Input: part model. Units: mm. Frame: model coordinates. Face numbers are marked on the shaded views. A direction names the side the tool comes from. Round coordinates to 2 decimals unless told otherwise and drop trailing zeros. Order: outer loops, then holes, each group sorted by start corner. A loop starts at its lowest first (then second) coordinate and runs counter-clockwise, first axis right, second up. Notation, with made-up numbers: (34, 55.5) -> (87, 55.5) arc R18 ccw to (87, 79.5) -> close; hole circle Ø5 at (-15, 30). An arc over 180 degrees is marked (long way). Answer as CSV lines item,"result". Start each with the question number.
1) First-contact query: P1, Ø1.2, axis at x = -6, z = -10.5, coming from the -Y side; P2, Ø2.5, axis at y = 9.5, z = -6, coming from the +X side; P3, Ø1, axis at x = -3.5, y = -1, coming from the -Z side. Flat tips, straight axial feed; report the tip coordinate or a pass-through.
2) Section query D-D, the plane z = 0.5. Output: boundary loops of the cut face in (x, y).
3) Access query for the marked faces 5 and 6. Directions: +Z, -Z, +X, -X, +Y, -Y. A direction counts if a zero-diameter tool reaches every point of the face in a straight line with its end or side. Return the directions, or none.
4) Section query B-B, the plane z = 6.5. Output: boundary loops of the cut face in (x, y), and give its area (3 significant figures).
5) Section query A-A, the plane z = 9. Output: boundary loops of the cut face in (x, y), and give its area (3 significant figures).
6) Section query C-C, the plane x = 7. Output: boundary loops of the cut face in (y, z), and give its area (3 significant figures).
7) Mould query, pull axis Z, two halves, no side actions, for the marked faces 1, 2, 3 and 4. Classes: +Z half, -Z half, draft (parallel to the pull), parting line (faces both ways), or undercut.
8) Line query: L1, parallel to Z at x = -13.9, y = 10; L2, parallel to X at y = 6.25, z = 3.75; L3, parallel to Z at x = -10.5, y = -0.75. Output: solid intervals per line, ascending.
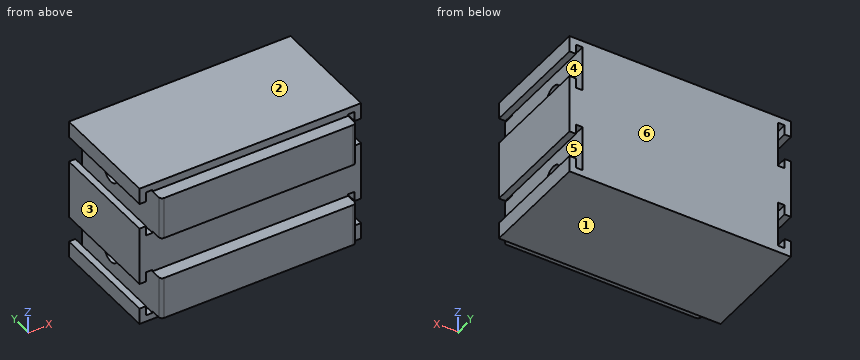
```python
from build123d import *

# Parameters (mm, degrees)
F0_W      = 34
F0_H      = 22
F1_DEPTH  = 17
F3_DEPTH  = 17.001
F4_W      = 30
F4_H      = 6.5
F5_DEPTH  = 2
F7_R      = 1.6
F8_DEPTH  = 5
F10_R     = 1.6
F11_DEPTH = 5
F12_R     = 0.5


with BuildPart() as f1:
    # F0 (on Front) → F1 (new body)
    with BuildSketch(Plane.XZ):
        Rectangle(F0_W, F0_H)
    extrude(amount=-F1_DEPTH)

    # F2 (on face) → F3 (cut, through all)
    with BuildSketch(Plane.XZ):
        Polygon((-16, 8.5), (-17, 8.5), (-17, 4.5), (-16, 4.5), (-16, 3), (-15, 3), (-15, 10), (-16, 10), align=None)
        Polygon((15, 10), (15, 3), (16, 3), (16, 4.5), (17, 4.5), (17, 8.5), (16, 8.5), (16, 10), align=None)
        Polygon((17, -4.5), (16, -4.5), (16, -3), (15, -3), (15, -10), (16, -10), (16, -8.5), (17, -8.5), align=None)
        Polygon((-17, -4.5), (-17, -8.5), (-16, -8.5), (-16, -10), (-15, -10), (-15, -3), (-16, -3), (-16, -4.5), align=None)
    extrude(amount=-F3_DEPTH, mode=Mode.SUBTRACT)

    # F4 (on face) → F5 (join)
    with BuildSketch(Plane.XZ):
        with Locations((0, 6.5)):
            Rectangle(F4_W, F4_H)
        with Locations((0, -6.5)):
            Rectangle(F4_W, F4_H)
    extrude(amount=F5_DEPTH)

    # F7 (on offset) → F8 (cut)
    with BuildSketch(Plane(origin=(-15, 0, 0), x_dir=(0, -1, 0), z_dir=(-1, 0, 0))):
        with Locations((-10, 6.5)):
            Circle(F7_R)
        with Locations((-10, -6.5)):
            Circle(F7_R)
    extrude(amount=-F8_DEPTH, mode=Mode.SUBTRACT)

    # F10 (on offset) → F11 (cut)
    with BuildSketch(Plane.YZ.offset(15)):
        with Locations((10, 6.5)):
            Circle(F10_R)
        with Locations((10, -6.5)):
            Circle(F10_R)
    extrude(amount=-F11_DEPTH, mode=Mode.SUBTRACT)

    # F12
    f12_edges = [f1.edges().sort_by_distance(p)[0] for p in [
        (15, -2, 6.5),
        (-15, -2, 6.5),
        (15, -2, -6.5),
        (-15, -2, -6.5),
    ]]
    fillet(f12_edges, radius=F12_R)


solid = f1.part
```
Findings:
1,P1,"stops at y = 0"
1,P2,"stops at x = 15"
1,P3,"stops at z = -9.75"
2,outline,"(-17, 0) -> (17, 0) -> (17, 17) -> (-17, 17) -> close"
3,face 5,"+Y, -Y"
3,face 6,"+Z, -Z, +X, -X, +Y"
4,outline,"(-15, -1.5) arc R0.5 ccw to (-14.5, -2) -> (14.5, -2) arc R0.5 ccw to (15, -1.5) -> (15, 8.4) -> (10, 8.4) -> (10, 11.6) -> (15, 11.6) -> (15, 17) -> (-15, 17) -> (-15, 11.6) -> (-10, 11.6) -> (-10, 8.4) -> (-15, 8.4) -> close"
4,area,"538 mm^2"
5,outline,"(-17, 0) -> (-16, 0) -> (-16, 17) -> (-17, 17) -> close; (-15, -1.5) arc R0.5 ccw to (-14.5, -2) -> (14.5, -2) arc R0.5 ccw to (15, -1.5) -> (15, 17) -> (-15, 17) -> close; (16, 0) -> (17, 0) -> (17, 17) -> (16, 17) -> close"
5,area,"604 mm^2"
6,outline,"(-2, -9.75) -> (0, -9.75) -> (0, -11) -> (17, -11) -> (17, 11) -> (0, 11) -> (0, 9.75) -> (-2, 9.75) -> (-2, 3.25) -> (0, 3.25) -> (0, -3.25) -> (-2, -3.25) -> close"
6,area,"400 mm^2"
7,face 1,"-Z half"
7,face 2,"+Z half"
7,face 3,"draft"
7,face 4,"undercut"
8,L1,"z = -11 to -8.1, -4.9 to 4.9, 8.1 to 11"
8,L2,"x = -17 to -16, -15 to 15, 16 to 17"
8,L3,"z = -9.75 to -3.25, 3.25 to 9.75"
